```python
from build123d import *

# Parameters (mm, degrees)
SKETCH1_R           = 9
SKETCH1_R_2         = 2.1
BOSS_EXTRUDE1_DEPTH = 4
SKETCH2_R           = 2.1
CUT_EXTRUDE1_DEPTH  = 183.748067126


with BuildPart() as part:
    # Sketch1 → Boss-Extrude1 (new body)
    with BuildSketch(Plane.XY):
        with BuildLine():
            Line((-116.359993818, -109.359993818), (116.359993818, -109.359993818))
            ThreePointArc((116.359993818, -109.359993818), (137.573197254, -100.573197254), (146.359993818, -79.359993818))
            Line((146.359993818, -79.359993818), (146.359993818, 79.359993818))
            ThreePointArc((146.359993818, 79.359993818), (137.573197254, 100.573197254), (116.359993818, 109.359993818))
            Line((116.359993818, 109.359993818), (-116.359993818, 109.359993818))
            ThreePointArc((-116.359993818, 109.359993818), (-137.573197254, 100.573197254), (-146.359993818, 79.359993818))
            Line((-146.359993818, 79.359993818), (-146.359993818, -79.359993818))
            ThreePointArc((-146.359993818, -79.359993818), (-137.573197254, -100.573197254), (-116.359993818, -109.359993818))
        make_face()
        with Locations((-101.359993818, -34.359993818)):
            Circle(SKETCH1_R, mode=Mode.SUBTRACT)
        with Locations((101.359993818, -34.359993818)):
            Circle(SKETCH1_R, mode=Mode.SUBTRACT)
        with Locations((-98.375, 71.25)):
            Circle(SKETCH1_R_2, mode=Mode.SUBTRACT)
        with Locations((98.375, 71.25)):
            Circle(SKETCH1_R_2, mode=Mode.SUBTRACT)
        with Locations((98.375, -71.25)):
            Circle(SKETCH1_R_2, mode=Mode.SUBTRACT)
        with Locations((-98.375, -71.25)):
            Circle(SKETCH1_R_2, mode=Mode.SUBTRACT)
    extrude(amount=BOSS_EXTRUDE1_DEPTH)

    # Sketch2 → Cut-Extrude1 (cut, through all)
    with BuildSketch(Plane.XY.offset(4)):
        with Locations((-70.359993818, 74.659993818)):
            Circle(SKETCH2_R)
        with Locations((-70.359993818, 19.659993818)):
            Circle(SKETCH2_R)
        with Locations((31.859993818, 74.659993818)):
            Circle(SKETCH2_R)
        with Locations((31.859993818, 19.659993818)):
            Circle(SKETCH2_R)
    extrude(amount=-CUT_EXTRUDE1_DEPTH, mode=Mode.SUBTRACT)


solid = part.part
```
CAD build for the part. Positions are in the model's coordinates, mm. Round coordinates to 2 decimals unless told otherwise and drop trailing zeros. Answer as CSV lines item,"result". Start each with the question number.
1. Pull direction X, two halves, no side cores. Call faces 1 (the face through (137.805, 100.339, 1.972)), 2 (the face through (-2, 2, 4)), 3 (the face through (109.944, -31.657, 1.972)): +X half, -X half, draft (parallel to the pull), parting line (faces both ways), or undercut.
2. Drill centre lines: L1, parallel to Y at x = 100, z = 3.4; L2, parallel to Y at x = 32.5, z = 3.4; L3, parallel to X at y = 74, z = 2.3. Where is each one in solid material? Low to high. Write a range as [from, to].
3. Saw through at A-A, the plane z = 1.8. Count the separate pieces of the cut face and the enclosed holes in it, and give its area (3 significant figures).
4. Pin check, flat tip, straight feed: pin 1 (2.5 mm diameter, centred on x = 31.86, y = 74.66, fed in from +Z). Stop position of the tip, or through.
Model answer:
1,face 1,"+X half"
1,face 2,"draft"
1,face 3,"undercut"
2,L1,"y = [-109.36, -72.58], [-69.92, -43.26], [-25.46, 69.92], [72.58, 109.36]"
2,L2,"y = [-109.36, 17.66], [21.66, 72.66], [76.66, 109.36]"
2,L3,"x = [-146.36, -72.35], [-68.37, 29.87], [33.85, 146.36]"
3,separate pieces,"1"
3,enclosed holes,"10"
3,area,"62,600 mm²"
4,pin 1,"passes through"
